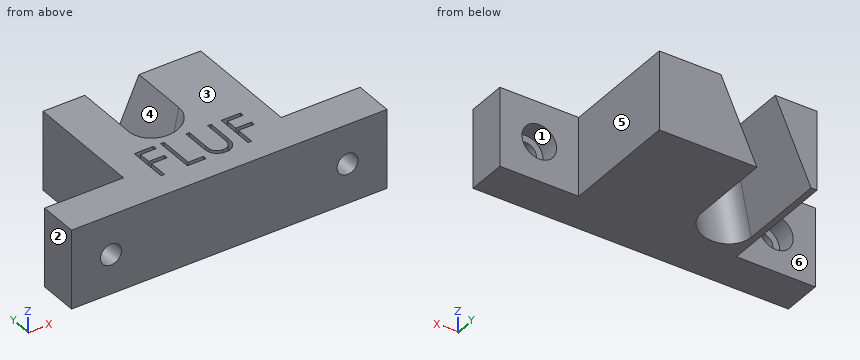
```python
from build123d import *

# Parameters (mm, degrees)
BOSS_EXTRUDE1_DEPTH                              = 25.4
CBORE_FOR_1_4_SOCKET_HEAD_CAP_SCREW1_D           = 6.7564
CBORE_FOR_1_4_SOCKET_HEAD_CAP_SCREW1_CBORE_D     = 11.1125
CBORE_FOR_1_4_SOCKET_HEAD_CAP_SCREW1_CBORE_DEPTH = 6.35
SKETCH6_R                                        = 7.9375
CUT_EXTRUDE2_DEPTH                               = 88.530033839
CUT_EXTRUDE3_DEPTH                               = 3.175


with BuildPart() as part:
    # Sketch1 → Boss-Extrude1 (new body)
    with BuildSketch(Plane.XY):
        Polygon((25.4, 12.7), (50.8, 12.7), (50.8, 0), (-50.8, 0), (-50.8, 12.7), (-25.4, 12.7), (-25.4, 50.8), (25.4, 50.8), align=None)
    extrude(amount=BOSS_EXTRUDE1_DEPTH)

    # CBORE for 1/4 Socket Head Cap Screw1 (through all)
    with Locations(Plane(origin=(0, 12.7, 0), x_dir=(1, 0, 0), z_dir=(0, 1, 0))):
        with Locations((-38.1, -12.7), (38.1, -12.7)):
            CounterBoreHole(CBORE_FOR_1_4_SOCKET_HEAD_CAP_SCREW1_D / 2, CBORE_FOR_1_4_SOCKET_HEAD_CAP_SCREW1_CBORE_D / 2, CBORE_FOR_1_4_SOCKET_HEAD_CAP_SCREW1_CBORE_DEPTH)

    # Sketch6 → Cut-Extrude2 (cut, through all)
    with BuildSketch(Plane(origin=(8.61013147, 38.672281651, 51.345863849), x_dir=(-0.9161407044196058, 0.08766347581543056, 0.39115383765662576), z_dir=(-0.40011338654688333, -0.2593820230581922, -0.878993881673942))):
        Circle(SKETCH6_R)
        with BuildLine():
            Line((-4.081369276, 42.668005296), (-7.904732998, 0.720487673))
            ThreePointArc((-7.904732998, 0.720487673), (0.360616196, 7.929304018), (7.9375, 0))
            ThreePointArc((7.9375, 0), (7.929304018, -0.360616196), (7.904732998, -0.720487673))
            Line((7.904732998, -0.720487673), (11.728096719, 41.227029949))
            Line((11.728096719, 41.227029949), (-4.081369276, 42.668005296))
        make_face()
    extrude(amount=CUT_EXTRUDE2_DEPTH, mode=Mode.SUBTRACT)

    # Sketch7 → Cut-Extrude3 (cut)
    with BuildSketch(Plane.XY.offset(25.4)):
        Polygon((-16.614726636, 20.539659198), (-10.427547149, 20.539659198), (-10.427547149, 19.237095095), (-15.474983047, 19.237095095), (-15.474983047, 15.329402787), (-10.427547149, 15.329402787), (-10.427547149, 14.026838685), (-15.474983047, 14.026838685), (-15.474983047, 7.839659198), (-16.614726636, 7.839659198), align=None)
        Polygon((-8.14805997, 20.539659198), (-7.00831638, 20.539659198), (-7.00831638, 9.1422233), (-2.123700995, 9.1422233), (-2.123700995, 7.839659198), (-8.14805997, 7.839659198), align=None)
        with BuildLine():
            Line((-0.007034329, 20.539659198), (1.132709261, 20.539659198))
            Line((1.132709261, 20.539659198), (1.132709261, 12.930344294))
            add(Edge.make_bspline(
                [(1.132709261, 12.930344294), (1.132539647, 12.822645624), (1.132217776, 12.618268839), (1.134367755, 12.327372434), (1.140388891, 12.068755225), (1.144184956, 11.841420336), (1.152629852, 11.646410938), (1.159517051, 11.482670525), (1.168372785, 11.350974419), (1.179015812, 11.274117916), (1.183590671, 11.241081473)],
                knots=[0, 0, 0, 0, 1.528628734, 2.90083645, 4.128790002, 5.200304208, 6.127813768, 6.898992206, 7.526736466, 8, 8, 8, 8], degree=3))
            add(Edge.make_bspline(
                [(1.183590671, 11.241081473), (1.20237745, 11.121894646), (1.238892441, 10.890236743), (1.331952154, 10.560369549), (1.461918515, 10.263075401), (1.615926127, 9.989077287), (1.818881603, 9.746001609), (2.062008717, 9.522076469), (2.356568048, 9.326235921), (2.684085103, 9.147162975), (3.037091536, 9.003235391), (3.397812417, 8.894402326), (3.760825513, 8.828076032), (4.003853312, 8.820396019), (4.124536184, 8.816582275)],
                knots=[0, 0, 0, 0, 1.035780045, 2.013197591, 2.933192213, 3.817615948, 4.702609284, 5.640816605, 6.646850145, 7.73207398, 8.84249596, 9.914020372, 10.964143139, 12, 12, 12, 12], degree=3))
            add(Edge.make_bspline(
                [(4.124536184, 8.816582275), (4.228145471, 8.820478817), (4.434765624, 8.828249397), (4.741766101, 8.876369446), (5.040760781, 8.963094356), (5.333226105, 9.074998622), (5.607368249, 9.222854167), (5.863340167, 9.39365407), (6.0918093, 9.593990678), (6.300299749, 9.815697642), (6.481855087, 10.065850631), (6.639230373, 10.339002731), (6.768138746, 10.639264647), (6.831796679, 10.850282122), (6.864500126, 10.958689646)],
                knots=[0, 0, 0, 0, 0.994687771, 1.983630487, 2.973142513, 3.978332533, 4.983357753, 5.956394766, 6.925816176, 7.893390482, 8.871859704, 9.88551698, 10.913711441, 12, 12, 12, 12], degree=3))
            add(Edge.make_bspline(
                [(6.864500126, 10.958689646), (6.875386295, 11.00349733), (6.899645067, 11.103346908), (6.922312916, 11.272152734), (6.945922308, 11.471322711), (6.962303748, 11.702287861), (6.97827389, 11.964274247), (6.987828183, 12.258646667), (6.992244274, 12.584336211), (6.993560286, 12.811619626), (6.994247723, 12.930344294)],
                knots=[0, 0, 0, 0, 0.558680831, 1.244966039, 2.062412453, 2.990489873, 4.051219941, 5.244515665, 6.560634259, 8, 8, 8, 8], degree=3))
            Line((6.994247723, 12.930344294), (6.994247723, 20.539659198))
            Line((6.994247723, 20.539659198), (8.133991312, 20.539659198))
            Line((8.133991312, 20.539659198), (8.133991312, 12.869286602))
            add(Edge.make_bspline(
                [(8.133991312, 12.869286602), (8.133069218, 12.731043912), (8.131269696, 12.461254899), (8.115664747, 12.06591711), (8.090783633, 11.690893435), (8.055629714, 11.336133462), (8.009049731, 11.002906656), (7.957251074, 10.688292211), (7.89128534, 10.394548495), (7.814238427, 10.119385151), (7.726160124, 9.85745486), (7.612073671, 9.608866458), (7.483533343, 9.366062779), (7.331080174, 9.132716213), (7.1597703, 8.907793577), (6.965817058, 8.692658933), (6.755635103, 8.483874394), (6.525730415, 8.286795554), (6.279892795, 8.106061212), (6.01885352, 7.947137871), (5.744617813, 7.812795031), (5.457898526, 7.702210962), (5.158573304, 7.619063702), (4.846634599, 7.55710528), (4.521372383, 7.5218998), (4.300157774, 7.516667654), (4.188137947, 7.514018172)],
                knots=[0, 0, 0, 0, 1.316592851, 2.569410997, 3.76748051, 4.895814652, 5.963796859, 6.97159953, 7.931736103, 8.829262218, 9.692595152, 10.560224239, 11.431080259, 12.30701507, 13.211635791, 14.121146779, 15.063487852, 16.031507147, 17.00238618, 17.966455255, 18.938106653, 19.907068911, 20.888905087, 21.893141452, 22.933117798, 24, 24, 24, 24], degree=3))
            add(Edge.make_bspline(
                [(4.188137947, 7.514018172), (4.065967203, 7.516865749), (3.826268641, 7.522452684), (3.473070511, 7.554466663), (3.134473285, 7.614767694), (2.806900816, 7.691548061), (2.494812841, 7.797443337), (2.194028057, 7.921170818), (1.909697986, 8.073125449), (1.637209948, 8.242192903), (1.383845832, 8.432419447), (1.151263827, 8.63975665), (0.939079954, 8.860883162), (0.750870684, 9.098193061), (0.58351776, 9.349840684), (0.439353843, 9.616537925), (0.3155715, 9.898181529), (0.251684814, 10.093954571), (0.219387947, 10.192924422)],
                knots=[0, 0, 0, 0, 1.13879206, 2.234305948, 3.301075583, 4.341971843, 5.366689343, 6.369221514, 7.369726634, 8.367512178, 9.355451585, 10.318319045, 11.268648973, 12.207971039, 13.137398894, 14.081662264, 15.030215811, 16, 16, 16, 16], degree=3))
            add(Edge.make_bspline(
                [(0.219387947, 10.192924422), (0.200602259, 10.260534049), (0.159855683, 10.407180837), (0.116221031, 10.649883238), (0.079539506, 10.929337368), (0.045047909, 11.245562354), (0.024695405, 11.598803299), (0.006852127, 11.988907079), (-0.007160032, 12.416345397), (-0.007077401, 12.714086068), (-0.007034329, 12.869286602)],
                knots=[0, 0, 0, 0, 0.625038921, 1.35572334, 2.194682327, 3.136881307, 4.189498639, 5.346923369, 6.617055217, 8, 8, 8, 8], degree=3))
            Line((-0.007034329, 12.869286602), (-0.007034329, 20.539659198))
        make_face()
        Polygon((11.390401569, 20.539659198), (17.577581056, 20.539659198), (17.577581056, 19.237095095), (12.530145158, 19.237095095), (12.530145158, 15.329402787), (17.577581056, 15.329402787), (17.577581056, 14.026838685), (12.530145158, 14.026838685), (12.530145158, 7.839659198), (11.390401569, 7.839659198), align=None)
    extrude(amount=-CUT_EXTRUDE3_DEPTH, mode=Mode.SUBTRACT)


solid = part.part
```
Geometry: final body of the model. Coordinates: model frame, mm. Face numbers are marked on the shaded views. A direction names the side the tool comes from. Round coordinates to 2 decimals unless told otherwise and drop trailing zeros. Loops run counter-clockwise (first coordinate to the right, second up) from the corner with the lowest first, then second, coordinate; pieces in that order, holes last. Notation, with made-up numbers: (9, 34) -> (38, 34) arc R15 ccw to (38, 46) -> close; hole circle Ø8 at (67.25, 64). An arc over 180 degrees is marked (long way). Use one line per item in the form item = value.
Item 1: Material intervals for probe 1 along X at (y, z) = (4.5, 12.7); probe 2 along Z at (x, y) = (38.1, 9); probe 3 along Z at (x, y) = (-38.1, 2.5), sorted ascending.
Evaluation:
probe_1 = -50.8 to -41.48, -34.72 to 34.72, 41.48 to 50.8
probe_2 = 0 to 7.14, 18.26 to 25.4
probe_3 = 0 to 9.32, 16.08 to 25.4
Item 2: Contact query for flat-ended pins moving along their axis: pin 1 Ø2 at (x, y) = (-27, 29) entering from -Z; pin 2 Ø9 at (x, z) = (38.5, 14) entering from +Y; pin 3 Ø6 at (y, z) = (35, 11.5) entering from -X; pin 4 Ø12.5 at (y, z) = (22.5, 12) entering from +X. Output: stop coordinate, or through.
Evaluation:
pin_1 = through
pin_2 = 12.7
pin_3 = -25.4
pin_4 = 25.4
Item 3: Cut plane C-C on z = 12.7. Give the number of separate pieces and of enclosed holes in the cut face, then the cut area to 3 significant figures.
Evaluation:
separate_pieces = 3
enclosed_holes = 0
area = 2,480 mm2
Item 4: Cut plane B-B on y = 46.5. Output: boundary loops of the cut face in (x, z), then the cut area to 3 significant figures.
Evaluation:
outline = (-25.4, 0) -> (-23.48, 0) -> (-11.92, 25.4) -> (-25.4, 25.4) -> close; (-6.04, 0) -> (25.4, 0) -> (25.4, 25.4) -> (5.52, 25.4) -> close
area = 847 mm2
Item 5: Draft query along X for the marked faces 1, 2 and 3. Return one class per face: released by +X, released by -X, zero draft, split by the parting line, or undercut.
Evaluation:
face_1 = undercut
face_2 = released by -X
face_3 = zero draft
Item 6: Cut plane A-A on x = -38.1. Output: boundary loops of the cut face in (y, z).
Evaluation:
outline = (0, 0) -> (12.7, 0) -> (12.7, 7.14) -> (6.35, 7.14) -> (6.35, 9.32) -> (0, 9.32) -> close; (0, 16.08) -> (6.35, 16.08) -> (6.35, 18.26) -> (12.7, 18.26) -> (12.7, 25.4) -> (0, 25.4) -> close
Item 7: Access query for the marked faces 4, 5 and 6. Directions: +Z, -Z, +X, -X, +Y, -Y. A direction counts if a zero-diameter tool reaches every point of the face in a straight line with its end or side. Return the directions, or none.
Evaluation:
face_4 = +Z, +Y
face_5 = +Z, -Z, +X, +Y
face_6 = +Z, -Z, -X, +Y
